Can you work these out from the drawing? Everything is in mm from the part's minimum corner. A direction names the side the tool comes from. Round coordinates to 2 decimals unless told otherwise and drop trailing zeros. Write each loop counter-clockwise with the first axis right and the second up, starting at its lowest first coordinate (ties: lowest second). Pieces come first, ordered by that corner, then holes. Notation, with made-up numbers: (25, 19) - (68, 19) arc R13 ccw to (68, 31) - close; hole circle Ø9 at (-18.5, 51.25). An arc over 180 degrees is marked (long way). One line per item, written item: value. Start each with the question number.
(1) Thinking about a two-plate mould opening in Y: for the marked faces 3, 4 and 5, which applies, +Y half, -Y half, draft (parallel to the pull), parting line (faces both ways), or undercut?
(2) I want a section at D-D on x = 5.5. List the corners of the cut face in (y, z) for me.
(3) I'm going to push flat-ended pins straight in: pin 1 Ø6 at (x, z) = (15, 8) entering from +Y; pin 2 Ø2 at (x, z) = (15, 8) entering from +Y; pin 3 Ø4.5 at (x, y) = (11, 11) entering from -Z; pin 4 Ø2 at (y, z) = (8, 8.5) entering from +X. Where does each tip first touch, or does it pass through?
(4) On a 3-axis mill with a long thin cutter (end or side, diameter ignored), from which of +Z, -Z, +X, -X, +Y, -Y can I reach the whole of each face in a straight line? I mean the marked faces 1 and 2. Say none if no direction works.
(5) I want a section at C-C on z = 6. List the corners of the cut face in (x, y) for me, plus the area to 3 significant figures.
(6) If I drill on L1, parallel to Y at x = 11, z = 9; L2, parallel to Z at x = 1.25, y = 15.25; L3, parallel to X at y = 8.75, z = 8.5, over which ranges is the centre line in solid material (lowest first)? Write a range as from..to.
(7) I want a section at A-A on y = 11. List the corners of the cut face in (x, z) for me.
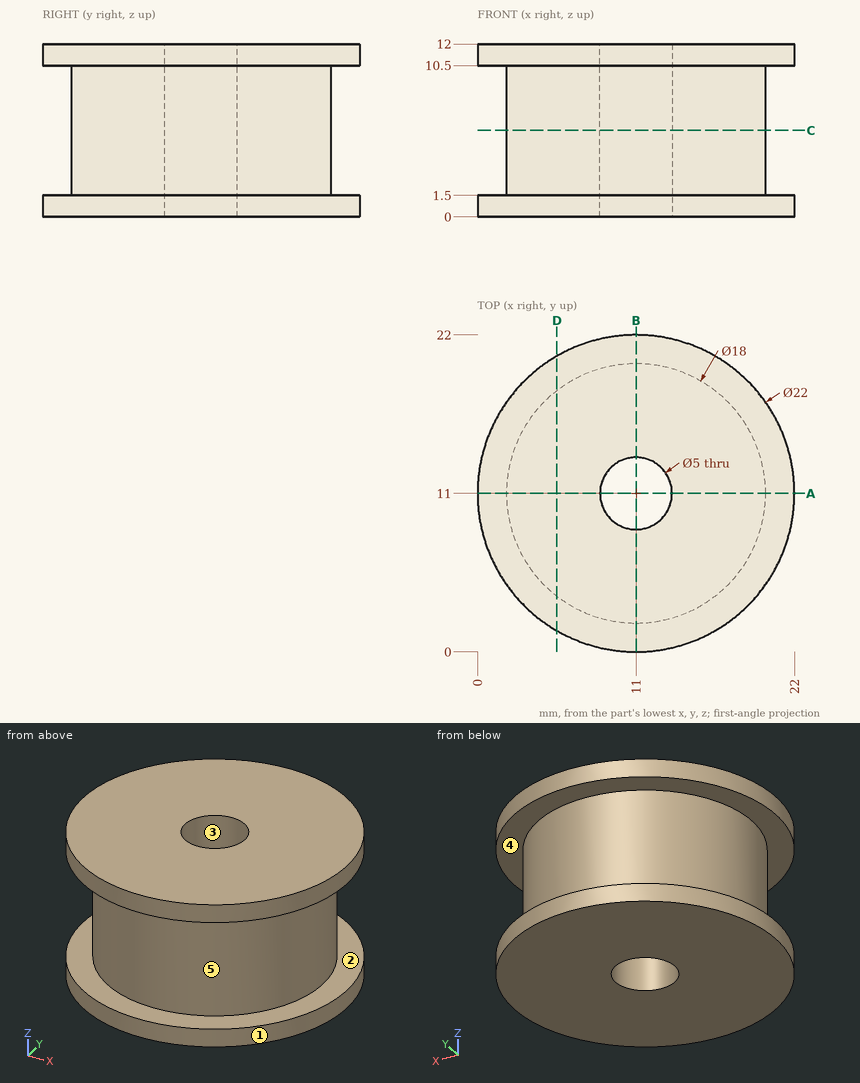
Established:
1. face 3: undercut
1. face 4: draft
1. face 5: parting line
2. outline: (1.47, 0) - (20.53, 0) - (20.53, 1.5) - (18.12, 1.5) - (18.12, 10.5) - (20.53, 10.5) - (20.53, 12) - (1.47, 12) - (1.47, 10.5) - (3.88, 10.5) - (3.88, 1.5) - (1.47, 1.5) - close
3. pin 1: y = 21.75
3. pin 2: y = 19.49
3. pin 3: through
3. pin 4: x = 19.77
4. face 1: +Z, -Z
4. face 2: none
5. outline: circle Ø18 at (11, 11); hole circle Ø5 at (11, 11)
5. area: 235 mm2
6. L1: 2..8.5, 13.5..20
6. L2: 0..1.5, 10.5..12
6. L3: 2.29..9.91, 12.09..19.71
7. outline: (0, 0) - (8.5, 0) - (8.5, 12) - (0, 12) - (0, 10.5) - (2, 10.5) - (2, 1.5) - (0, 1.5) - close; (13.5, 0) - (22, 0) - (22, 1.5) - (20, 1.5) - (20, 10.5) - (22, 10.5) - (22, 12) - (13.5, 12) - close
